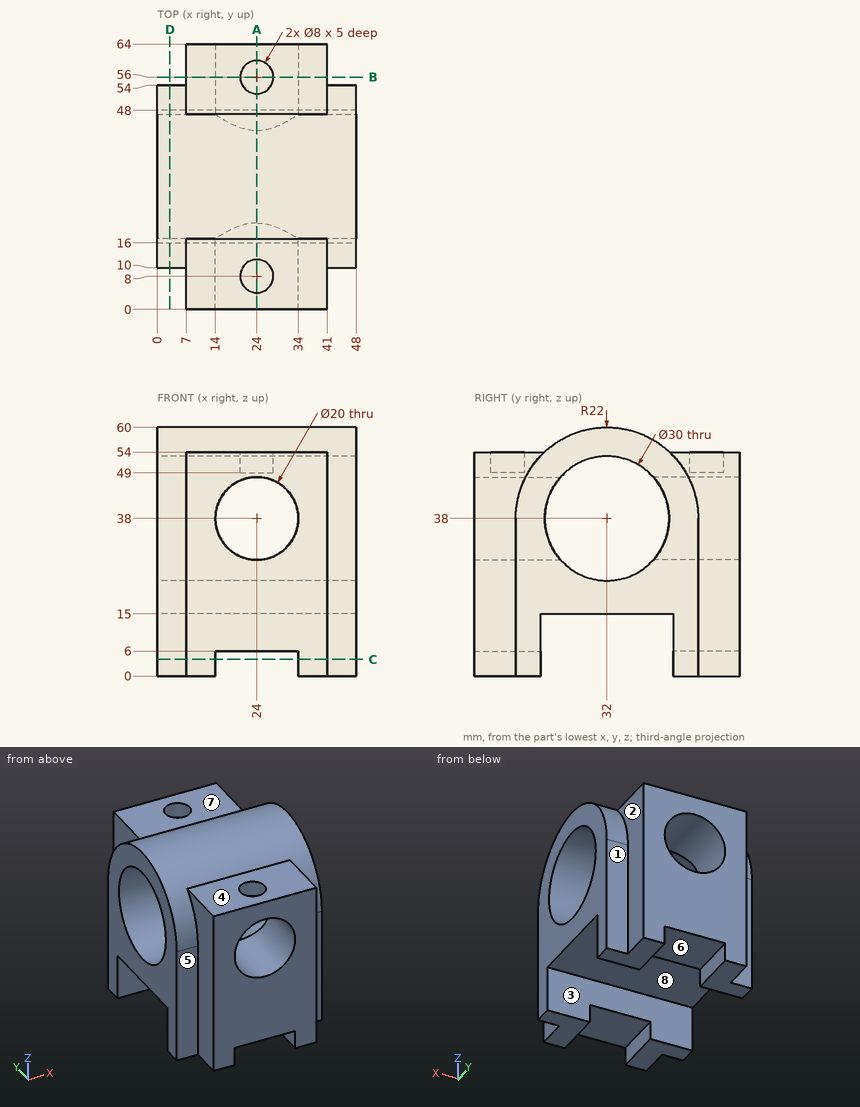
Study the drawing (mm; zero at the part's minimum x, y, z) and answer. A direction names the side the tool comes from. Round coordinates to 2 decimals unless told otherwise and drop trailing zeros. Loops run counter-clockwise (first coordinate to the right, second up) from the corner with the lowest first, then second, coordinate; pieces in that order, holes last. Notation, with made-up numbers: (-36.75, -13) -> (-0.75, -13) arc R17 ccw to (-0.75, -1) -> close; hole circle Ø2 at (32, 84). An arc over 180 degrees is marked (long way). Write each question's results on one line, items separated by ' | '. Start each with the question number.
1. Find the intervals of material crossed by probe 1 along X at (y, z) = (8, 52); probe 2 along Y at (x, z) = (5, 14); probe 3 along X at (y, z) = (48.5, 38), in increasing order. Write a range as from..to.
2. Section C-C (z = 4) is taken. Determine the outline of the cut face in (x, y), plus the area to 3 significant figures.
3. Section A-A (x = 24) is taken. Determine the outline of the cut face in (y, z).
4. A tool of negligible diameter and unlimited length cuts with its end or side. For the marked faces 4, 5, 6, 7 and 8, from which of +Z, -Z, +X, -X, +Y, -Y can it reach the whole face along a straight path? Write none if from no direction.
5. Section D-D (x = 3) is taken. Determine the outline of the cut face in (y, z), plus the area to 3 significant figures.
6. Section B-B (y = 56) is taken. Determine the outline of the cut face in (x, z).
7. For a pull along Y with two mould halves and no side action, classify the marked faces 1, 2 and 3 as +Y half, -Y half, draft (parallel to the pull), parting line (faces both ways), or undercut.
8. Given pin 1 Ø1.8 at (y, z) = (4.5, 3) entering from -X; pin 2 Ø2 at (x, z) = (43.5, 19) entering from +Y; pin 3 Ø12 at (y, z) = (28, 32) entering from +X; pin 4 Ø5 at (x, y) = (18, 55) entering from +Z, each flat-ended and moving along its own axis, determine where each tip first touches the part or whether it passes through.
Evaluation:
1) probe 1: x = 7..20, 28..41 | probe 2: y = 10..16, 48..54 | probe 3: x = 0..14, 34..48
2) outline: (0, 10) -> (7, 10) -> (7, 0) -> (14, 0) -> (14, 16) -> (0, 16) -> close; (0, 48) -> (14, 48) -> (14, 64) -> (7, 64) -> (7, 54) -> (0, 54) -> close; (34, 0) -> (41, 0) -> (41, 10) -> (48, 10) -> (48, 16) -> (34, 16) -> close; (34, 48) -> (48, 48) -> (48, 54) -> (41, 54) -> (41, 64) -> (34, 64) -> close | area: 616 mm2
3) outline: (0, 6) -> (16, 6) -> (16, 15) -> (48, 15) -> (48, 6) -> (64, 6) -> (64, 28) -> (43.18, 28) arc R15 cw to (20.82, 28) -> (0, 28) -> close; (0, 48) -> (20.82, 48) arc R15 cw to (43.18, 48) -> (64, 48) -> (64, 54) -> (60, 54) -> (60, 49) -> (52, 49) -> (52, 54) -> (47.1, 54) arc R22 ccw to (16.9, 54) -> (12, 54) -> (12, 49) -> (4, 49) -> (4, 54) -> (0, 54) -> close
4) face 4: +Z, +X, -X, -Y | face 5: +Z, -Z, -X, -Y | face 6: -Z, +Y, -Y | face 7: +Z, +X, -X, +Y | face 8: -Z, +X, -X
5) outline: (10, 0) -> (16, 0) -> (16, 15) -> (48, 15) -> (48, 0) -> (54, 0) -> (54, 38) arc R22 ccw to (10, 38) -> close; hole circle Ø30 at (32, 38) | area: 1,250 mm2
6) outline: (7, 0) -> (14, 0) -> (14, 6) -> (34, 6) -> (34, 0) -> (41, 0) -> (41, 54) -> (28, 54) -> (28, 49) -> (20, 49) -> (20, 54) -> (7, 54) -> close; hole circle Ø20 at (24, 38)
7) face 1: +Y half | face 2: draft | face 3: undercut
8) pin 1: stops at x = 7 | pin 2: stops at y = 54 | pin 3: passes through | pin 4: stops at z = 54
